from build123d import *

# Parameters (mm, degrees)
F_3_0_3_DIAMETER_HOLE1_D = 3
CHAMFER1_SIZE            = 1


with BuildPart() as part:
    # Sketch1 → Revolve1 (revolve)
    with BuildSketch(Plane(origin=(0, 0, 0), x_dir=(0, 0, -1), z_dir=(1, 0, 0)), mode=Mode.PRIVATE) as revolve1_sk:
        Polygon((0, 0), (0, 8.5), (1, 8.5), (1, 10.5), (13, 10.5), (13, 8.5), (14, 8.5), (14, 5.5), (3, 5.5), (3, 0), align=None)
    revolve(revolve1_sk.sketch.rotate(Axis((0, 0, 21.219054242), (0, 0, -1)), 180), axis=Axis((0, 0, 21.219054242), (0, 0, -1)))

    # Ø3.0 (3) Diameter Hole1 (through all)
    with Locations(Plane.XY):
        with Locations((0, 0)):
            Hole(F_3_0_3_DIAMETER_HOLE1_D / 2)

    # Chamfer1
    chamfer1_edges = [part.edges().sort_by_distance(p)[0] for p in [
        (0, 5.5, -14),
    ]]
    chamfer(chamfer1_edges, length=CHAMFER1_SIZE)


solid = part.part
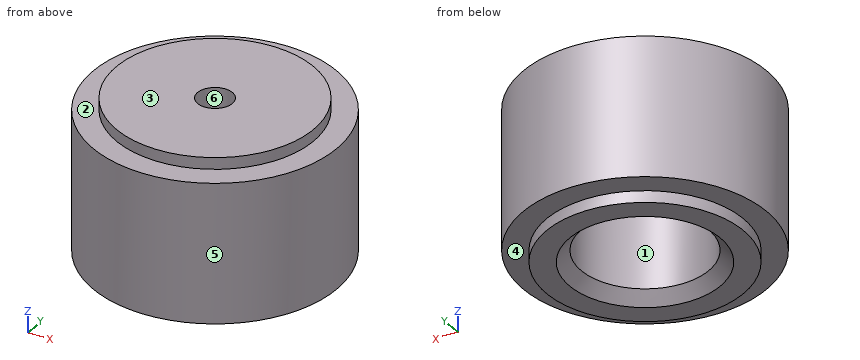
Source: CAD feature listing. Evaluate the final solid. Frame: model axes, mm. Face numbers are marked on the shaded views. A direction names the side the tool comes from. Give positions to 0.01 mm unless a question says otherwise; leave off trailing zeros. Write each loop counter-clockwise with the first axis right and the second up, starting at its lowest first coordinate (ties: lowest second). Pieces come first, ordered by that corner, then holes. Notation, with made-up numbers: (-27.5, 6.5) -> (0.5, 6.5) arc R24 cw to (0.5, 27.5) -> close; hole circle Ø4 at (5, 29.25). An arc over 180 degrees is marked (long way). Return JSON: item names as keys, results as strings. Group by question number.
1. Section A-A, the plane y = 0. Output: boundary loops of the cut face in (x, z).
2. Material intervals for line 1 (X direction, y = 0, z = -8.5); line 2 (Z direction, x = 9, y = -3.5); line 3 (Y direction, x = -1.75, z = -7.5), sorted ascending. Write a range as from..to.
3. Mould query, pull axis X, two halves, no side actions, for the marked faces 4, 5 and 6. Classes: +X half, -X half, draft (parallel to the pull), parting line (faces both ways), or undercut.
4. Section C-C, the plane z = -7.5. Output: boundary loops of the cut face in (x, y).
5. Access query for the marked faces 1, 2 and 3. Directions: +Z, -Z, +X, -X, +Y, -Y. A direction counts if a zero-diameter tool reaches every point of the face in a straight line with its end or side. Return the directions, or none.
6. Pin query (flat end, axial travel): pin 1 Ø3 at (y, z) = (-6.5, -10.5) entering from +X; pin 2 Ø6 at (y, z) = (4, -5.5) entering from +X; pin 3 Ø10 at (x, y) = (0, 0) entering from -Z. Return the tip coordinate at first contact, or that it passes through.
7. Section D-D, the plane x = 7. Output: boundary loops of the cut face in (y, z), then the cut area to 3 significant figures.
Determined:
{
 "1": {"outline": "(-10.5, -13) -> (-8.5, -13) -> (-8.5, -14) -> (-6.5, -14) -> (-5.5, -13) -> (-5.5, -3) -> (-1.5, -3) -> (-1.5, 0) -> (-8.5, 0) -> (-8.5, -1) -> (-10.5, -1) -> close; (1.5, -3) -> (5.5, -3) -> (5.5, -13) -> (6.5, -14) -> (8.5, -14) -> (8.5, -13) -> (10.5, -13) -> (10.5, -1) -> (8.5, -1) -> (8.5, 0) -> (1.5, 0) -> close"},
 "2": {"line 1": "x = -10.5..-5.5, 5.5..10.5", "line 2": "z = -13..-1", "line 3": "y = -10.35..-5.21, 5.21..10.35"},
 "3": {"face 4": "draft", "face 5": "parting line", "face 6": "undercut"},
 "4": {"outline": "circle Ø21 at (0, 0); hole circle Ø11 at (0, 0)"},
 "5": {"face 1": "-Z", "face 2": "+Z", "face 3": "+Z, +X, -X, +Y, -Y"},
 "6": {"pin 1": "stops at x = 9.23", "pin 2": "stops at x = 10.45", "pin 3": "stops at z = -3"},
 "7": {"outline": "(-7.83, -13) -> (-4.82, -13) -> (-4.82, -14) -> (4.82, -14) -> (4.82, -13) -> (7.83, -13) -> (7.83, -1) -> (4.82, -1) -> (4.82, 0) -> (-4.82, 0) -> (-4.82, -1) -> (-7.83, -1) -> close", "area": "207 mm2"}
}
